from build123d import *

# Parameters (mm, degrees)
SKETCH_1_R      = 1.5
EXTRUDE_1_DEPTH = 6
EXTRUDE_2_DEPTH = 30


with BuildPart() as part:
    # 草图1 → 凸台-拉伸1 (new body)
    with BuildSketch(Plane.XY):
        Circle(SKETCH_1_R)
    extrude(amount=EXTRUDE_1_DEPTH)

    # 草图2 → 凸台-拉伸2 (add)
    with BuildSketch(Plane(origin=(0, 0, 0), x_dir=(-1, 0, 0), z_dir=(0, 0, -1))):
        Polygon((1.456280061, -1.49922127), (2.026503736, 0.511564893), (0.570223675, 2.010786163), (-1.456280061, 1.49922127), (-2.026503736, -0.511564893), (-0.570223675, -2.010786163), align=None)
    extrude(amount=EXTRUDE_2_DEPTH)


solid = part.part
Work out the finished part from the listing and answer in its coordinate system (mm). A direction names the side the tool comes from. Round coordinates to 2 decimals unless told otherwise and drop trailing zeros. Order: outer loops, then holes, each group sorted by start corner. A loop starts at its lowest first (then second) coordinate and runs counter-clockwise, first axis right, second up. Notation, with made-up numbers: M 2.25,5 L 36.25,5 A21 cw 36.25,27 Z; hole C 23.25,41 d8. An arc over 180 degrees is marked long. Put each result on its own line as item: value. Start each with the question number.
Q1. Straight lines are drawn through the part: L1, parallel to Z at x = 1.05, y = 1.35; L2, parallel to Y at x = -1.1, z = -4.5; L3, parallel to Y at x = 0.15, z = -5. For each, find the intervals that lie inside material, in ascending order. Write a range as [from, to].
Q2. Section A-A, the plane z = -21 is taken. Write down the section's boundary in (x, y), and give its area (3 significant figures).
Q3. Section C-C, the plane y = 1 is taken. Write down the section's boundary in (x, z).
Q4. Section D-D, the plane z = 3.5 is taken. Write down the section's boundary in (x, y).
Q5. A tool of negligible diameter and unlimited length cuts with its end or side. For faces 1 (the flat face through (-1.31, 1.25, -14.79)), 2 (the cylindrical face through (-1.5, 0.07, 2.96)), from which of +Z, -Z, +X, -X, +Y, -Y can it reach the whole face along a straight path? Write none if from no direction.
Q6. Flat-ended cylindrical pins translate along their axes: pin 1 (1 mm diameter, centred on y = 0, z = -21, fed in from -X); pin 2 (2 mm diameter, centred on x = -1.5, y = 0.5, fed in from +Z). Find the tip coordinate at first contact, or state that the pin passes through.
Q7. Section B-B, the plane x = 0 is taken. Write down the section's boundary in (y, z), and give its area (3 significant figures).
Findings below:
1. L1: z = [-30, 0]
1. L2: y = [-1.59, 1.47]
1. L3: y = [-1.9, 1.83]
2. outline: M -2.03,0.51 L -1.46,-1.5 L 0.57,-2.01 L 2.03,-0.51 L 1.46,1.5 L -0.57,2.01 Z
2. area: 11.3 mm^2
3. outline: M -1.55,-30 L 1.6,-30 L 1.6,0 L 1.12,0 L 1.12,6 L -1.12,6 L -1.12,0 L -1.55,0 Z
4. outline: C 0,0 d3
5. face 1: +Z, -Z, -X, +Y
5. face 2: +Z
6. pin 1: stops at x = -2.02
6. pin 2: stops at z = 6
7. outline: M -1.87,-30 L 1.87,-30 L 1.87,0 L 1.5,0 L 1.5,6 L -1.5,6 L -1.5,0 L -1.87,0 Z
7. area: 130 mm^2
